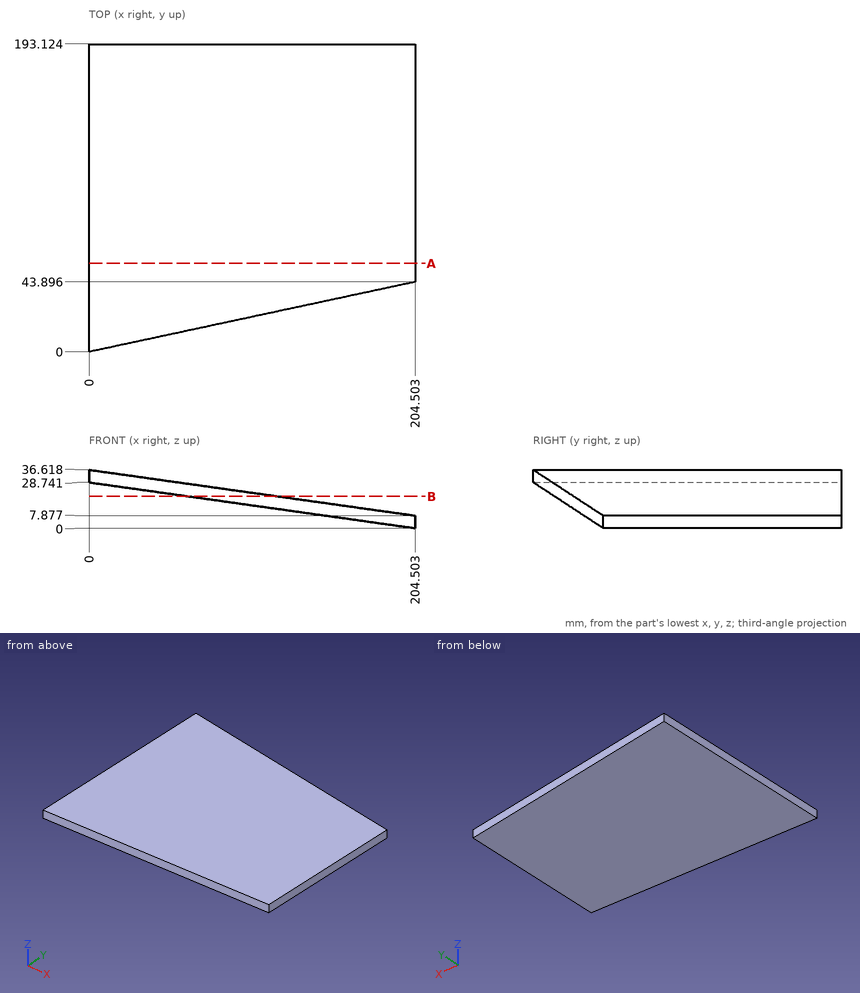
Part print with two shaded views. Sizes in mm from the minimum x, y, z corner. Coordinates: 2 decimals unless noted, no trailing zeros. Write each loop counter-clockwise with the first axis right and the second up, starting at its lowest first coordinate (ties: lowest second). Pieces come first, ordered by that corner, then holes. Notation, with made-up numbers: (70, -19.75) -> (118, -19.75) arc R9 cw to (118, -15.75) -> close; hole circle Ø10 at (-27, 39.25). An arc over 180 degrees is marked (long way). Return JSON: item names as keys, results as strings. Group by question number.
Q1. Flat gauge pins, fed straight in: pin 1 (3 mm diameter, centred on x = 105.5, z = 19.5, fed in from -Y); pin 2 (12 mm diameter, centred on x = 155, z = 7, fed in from -Y); pin 3 (6 mm diameter, centred on x = 50, y = 57.5, fed in from +Z). Where does each tip first touch, or does it go through?
Q2. Cut at A-A, the plane y = 55.5. Give the cut face in (x, z), then the cut area to 3 significant figures.
Q3. Drill centre lines: line 1 (Z direction, x = 56, y = 95); line 2 (Y direction, x = 128, z = 16.5) (1 decimal); line 3 (Y direction, x = 176.5, z = 7) (1 decimal). Where is each one in solid material? Low to high.
Q4. Cut at B-B, the plane z = 20. Give the cut face in (x, y).
Returned:
{
 "1": {"pin 1": "stops at y = 22.32", "pin 2": "stops at y = 31.99", "pin 3": "stops at z = 30.01"},
 "2": {"outline": "(0, 28.74) -> (204.5, 0) -> (204.5, 7.88) -> (0, 36.62) -> close", "area": "1,610 mm2"},
 "3": {"line 1": "z = 20.87 to 28.75", "line 2": "y = 27.5 to 193.1", "line 3": "y = 37.9 to 193.1"},
 "4": {"outline": "(62.2, 13.35) -> (118.24, 25.38) -> (118.24, 193.12) -> (62.2, 193.12) -> close"}
}
